Could you check a few things on this model? Use its own coordinates, in mm. A direction names the side the tool comes from. Coordinates: 2 decimals unless noted, no trailing zeros. Order: outer loops, then holes, each group sorted by start corner. A loop starts at its lowest first (then second) coordinate and runs counter-clockwise, first axis right, second up. Notation, with made-up numbers: (-38.5, 80.25) -> (10.5, 80.25) arc R19 ccw to (10.5, 103.25) -> close; hole circle Ø9 at (54, 57.25). An arc over 180 degrees is marked (long way). Use a Markdown table: item, result. Add a question column.
1) If we section it at D-D (y = 0.5): Write out the boundary of the cut face in (x, z), plus the area to 3 significant figures.
2) If we section it at C-C (x = 25): Write out the boundary of the cut face in (y, z).
3) Which directions (+Z, -Z, +X, -X, +Y, -Y) give clear straight access to the entire face, cutting with the end or side of a thin tool? Please do faces 4 (the flat face through (0, 1, 20)), 5 (the flat face through (-56, 40.5, 15)), 6 (the flat face through (60.8, 15, 7)), 7 (the flat face through (-50.8, 20, 7)), 8 (the cylindrical face through (-52.3, 17.71, 18.57)).
4) Will these pins go through, and if not, where does the flat tip stop? pin 1 Ø16.5 at (y, z) = (6.5, 8.5) entering from -X; pin 2 Ø12 at (x, y) = (-55.5, 7) entering from +Z; pin 3 Ø16.5 at (y, z) = (24, 10) entering from +X; pin 4 Ø5 at (x, y) = (-46, 26.5) entering from -Z.
5) Thinking about a two-plate mould opening in X: for faces 1 (the cylindrical face through (-59.37, -6, 7.61)), 2 (the cylindrical face through (0.78, -6, 18.57)), 3 (the cylindrical face through (42.678, 38.295, 14.79)), which applies, +X half, -X half, draft (parallel to the pull), parting line (faces both ways), or undercut?
6) If we section it at B-B (z = 3): Write out the boundary of the cut face in (x, y).
7) If I drill on L1, parallel to X at y = 23, z = 4; L2, parallel to Z at x = 32.5, y = -2.5; L3, parallel to Y at x = 37.5, z = 13.5, over which ranges is the centre line in solid material (lowest first)? Write a range as [from, to].
```python
from build123d import *

# Parameters (mm, degrees)
F0_W        = 101.6
F0_H        = 15
F1_DEPTH    = 20
F2_W        = 30
F2_H        = 30
F3_DEPTH    = 3
F4_R        = 4.99999
F5_T1_DEPTH = 52.9128784748
F5_T3_DEPTH = 52.9128784748
F5_T5_DEPTH = 52.9128784748


# Not quite as in the source:
# - a fillet or chamfer that OpenCascade refuses, or shapes differently, is made with other operations: its cross-section is extruded or revolved along the edge and cut away or added
# - a fillet or chamfer is up to 0.001 mm smaller than in the source, because OpenCascade refuses the exact size
# - a feature of the source that left no trace in its solid (it failed there, or was rolled back) is left out


with BuildPart() as f1:
    # F0 (on Top) → F1 (new body)
    with BuildSketch(Plane.XY):
        Rectangle(F0_W, F0_H)
        Polygon((50.8, 7.5), (50.8, -7.5), (60.8, -7.5), (60.8, 37.5), (50.8, 37.5), align=None)
        Polygon((-60.8, -7.5), (-50.8, -7.5), (-50.8, 7.5), (-50.8, 37.5), (-60.8, 37.5), align=None)
    extrude(amount=F1_DEPTH)

    # F2 (on face) → F3 (join)
    with BuildSketch(Plane(origin=(0, 37.5, 0), x_dir=(-1, 0, 0), z_dir=(0, 1, 0))):
        with Locations((-55.8, 15)):
            Rectangle(F2_W, F2_H)
        with Locations((55.8, 15)):
            Rectangle(F2_W, F2_H)
    extrude(amount=F3_DEPTH)

    # F4 (radius 5 in the source; OpenCascade refuses exactly that, so slightly less here)
    f4_edges = [f1.edges().sort_by_distance(p)[0] for p in [
        (-55.8, 37.5, 20),
        (-50.8, 37.5, 10),
        (-60.8, 37.5, 10),
        (-60.8, -7.5, 10),
        (60.8, -7.5, 10),
        (60.8, 37.5, 10),
        (55.8, 37.5, 20),
        (50.8, 37.5, 10),
        (60.8, 15, 20),
        (50.8, 22.5, 20),
        (0, 7.5, 20),
        (-50.8, 22.5, 20),
        (-60.8, 15, 20),
        (0, -7.5, 20),
    ]]
    fillet(f4_edges, radius=F4_R)

    # F5: fillet of radius 5 on 6 edges, made by hand

    # F5_s2 → F5_t1 (cut)
    with BuildSketch(Plane.YZ.offset(-82.2564392374)):
        with BuildLine():
            ThreePointArc((37.5, 25.417424305), (38.3166998673, 28.1560370926), (40.5, 30))
            Line((40.5, 30), (37.5, 30))
            Line((37.5, 30), (37.5, 25.417424305))
        make_face()
    extrude(amount=F5_T1_DEPTH, mode=Mode.SUBTRACT)

    # F5_s4 → F5_t3 (cut)
    with BuildSketch(Plane.XY.offset(-11.4564392374)):
        with BuildLine():
            ThreePointArc((-66.217424305, 37.5), (-68.9560370926, 38.3166998673), (-70.8, 40.5))
            Line((-70.8, 40.5), (-70.8, 37.5))
            Line((-70.8, 37.5), (-66.217424305, 37.5))
        make_face()
        with BuildLine():
            ThreePointArc((-45.382575695, 37.5), (-42.6439629074, 38.3166998673), (-40.8, 40.5))
            Line((-40.8, 40.5), (-40.8, 37.5))
            Line((-40.8, 37.5), (-45.382575695, 37.5))
        make_face()
        with BuildLine():
            ThreePointArc((45.382575695, 37.5), (42.6439629074, 38.3166998673), (40.8, 40.5))
            Line((40.8, 40.5), (40.8, 37.5))
            Line((40.8, 37.5), (45.382575695, 37.5))
        make_face()
        with BuildLine():
            ThreePointArc((66.217424305, 37.5), (68.9560370926, 38.3166998673), (70.8, 40.5))
            Line((70.8, 40.5), (70.8, 37.5))
            Line((70.8, 37.5), (66.217424305, 37.5))
        make_face()
    extrude(amount=F5_T3_DEPTH, mode=Mode.SUBTRACT)

    # F5_s6 → F5_t5 (cut)
    with BuildSketch(Plane.YZ.offset(29.3435607626)):
        with BuildLine():
            ThreePointArc((37.5, 25.417424305), (38.3166998673, 28.1560370926), (40.5, 30))
            Line((40.5, 30), (37.5, 30))
            Line((37.5, 30), (37.5, 25.417424305))
        make_face()
    extrude(amount=F5_T5_DEPTH, mode=Mode.SUBTRACT)


solid = f1.part
```
Answer sheet:
| question | item | result |
|---|---|---|
| 1 | outline | (-60.8, 0) -> (60.8, 0) -> (60.8, 15) arc R5 ccw to (55.8, 20) -> (-55.8, 20) arc R5 ccw to (-60.8, 15) -> close |
| 1 | area | 2,420 mm2 |
| 2 | outline | (-7.5, 0) -> (7.5, 0) -> (7.5, 15) arc R5 ccw to (2.5, 20) -> (-2.5, 20) arc R5 ccw to (-7.5, 15) -> close |
| 3 | face 4 | +Z, +X, -X, -Y |
| 3 | face 5 | +Z, -Z, +X, -X, +Y |
| 3 | face 6 | +Z, -Z, +X, -Y |
| 3 | face 7 | +Z, -Z |
| 3 | face 8 | +Z |
| 4 | pin 1 | x = -60.8 |
| 4 | pin 2 | z = 20 |
| 4 | pin 3 | x = 60.8 |
| 4 | pin 4 | through |
| 5 | face 1 | -X half |
| 5 | face 2 | draft |
| 5 | face 3 | undercut |
| 6 | outline | (-70.8, 40.5) arc R5 ccw to (-66.22, 37.5) -> (-65.8, 37.5) arc R5 cw to (-60.8, 32.5) -> (-60.8, -2.5) arc R5 ccw to (-55.8, -7.5) -> (55.8, -7.5) arc R5 ccw to (60.8, -2.5) -> (60.8, 32.5) arc R5 cw to (65.8, 37.5) -> (66.22, 37.5) arc R5 ccw to (70.8, 40.5) -> (40.8, 40.5) arc R5 ccw to (45.38, 37.5) -> (45.8, 37.5) arc R5 cw to (50.8, 32.5) -> (50.8, 7.5) -> (-50.8, 7.5) -> (-50.8, 32.5) arc R5 cw to (-45.8, 37.5) -> (-45.38, 37.5) arc R5 ccw to (-40.8, 40.5) -> close |
| 7 | L1 | [-60.8, -50.8], [50.8, 60.8] |
| 7 | L2 | [0, 20] |
| 7 | L3 | [-7.5, 7.5] |
